The figure shows three views and two pictorial views of one solid part (mm, origin at its lowest corner). Answer the questions. Round coordinates to 2 decimals unless told otherwise and drop trailing zeros. Order: outer loops, then holes, each group sorted by start corner. A loop starts at its lowest first (then second) coordinate and runs counter-clockwise, first axis right, second up. Notation, with made-up numbers: M 76,68 L 106,68 A22 cw 106,97 Z; hole C -11.5,85.5 d5. An arc over 180 degrees is marked long. Answer as CSV lines item,"result".
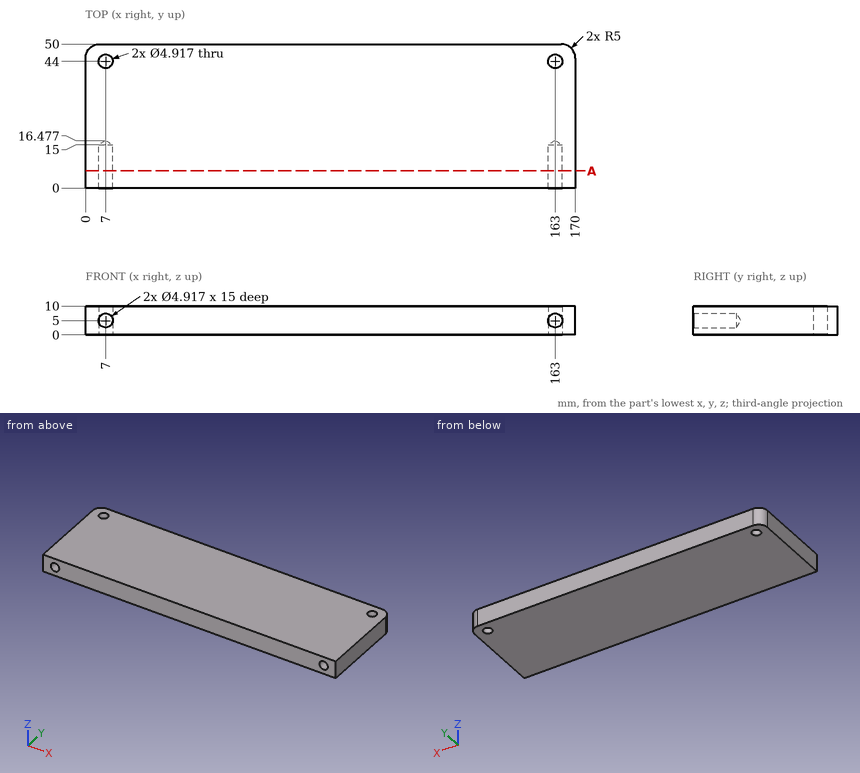
Item 1: A flat-ended cylindrical pin translates along its axis: pin 1 (4 mm diameter, centred on x = 163, y = 44, fed in from +Z). Find the tip coordinate at first contact, or state that the pin passes through.
Ans:
pin 1,"through"
Item 2: Find the intervals of material crossed by probe 1 along X at (y, z) = (4.75, 5); probe 2 along Z at (x, y) = (7, 10.5); probe 3 along Y at (x, z) = (8, 4.25), in increasing order. Write a range as [from, to].
Ans:
probe 1,"[0, 4.54], [9.46, 160.54], [165.46, 170]"
probe 2,"[0, 2.54], [7.46, 10]"
probe 3,"[15.73, 41.75], [46.25, 50]"
Item 3: A cutting plane is placed at A-A, the plane y = 6. Determine the outline of the cut face in (x, z).
Ans:
outline,"M 0,0 L 170,0 L 170,10 L 0,10 Z; hole C 7,5 d4.92; hole C 163,5 d4.92"
